```python
from build123d import *

# Parameters (mm, degrees)
F0_R     = 30.022303
F1_DEPTH = 10
F3_DEPTH = 25
F4_R     = 15.13861
F5_DEPTH = 25


with BuildPart() as f1:
    # F0 (on Front) → F1 (new body)
    with BuildSketch(Plane.XZ):
        Circle(F0_R)
    extrude(amount=F1_DEPTH)

    # F2 (on face) → F3 (cut)
    with BuildSketch(Plane.XZ.offset(10)):
        with BuildLine():
            ThreePointArc((-13.51767, 26.806926), (-0.223887, 30.021468), (13.11636, 27.005551))
            ThreePointArc((13.11636, 27.005551), (-0.226298, 30.344822), (-13.51767, 26.806926))
        make_face()
        with BuildLine():
            ThreePointArc((19.663822, -22.686401), (27.429863, -12.524318), (30.022303, 0))
            ThreePointArc((30.022303, 0), (27.31018, -12.469672), (19.663822, -22.686401))
        make_face()
        with BuildLine():
            ThreePointArc((-11.50515, -27.730312), (-22.127404, -20.290802), (-28.62096, -9.065281))
            ThreePointArc((-28.62096, -9.065281), (-22.573017, -20.699429), (-11.50515, -27.730312))
        make_face()
        with BuildLine():
            Line((-8.288842, 15.331867), (-13.51767, 26.806926))
            ThreePointArc((-13.51767, 26.806926), (-27.669836, 11.649842), (-28.62096, -9.065281))
            Line((-28.62096, -9.065281), (-16.901936, -3.498297))
            ThreePointArc((-16.901936, -3.498297), (-15.781932, 7.37434), (-8.288842, 15.331867))
        make_face()
        with BuildLine():
            ThreePointArc((-11.50515, -27.730312), (4.795961, -29.636758), (19.663822, -22.686401))
            Line((19.663822, -22.686401), (11.541307, -13.314021))
            ThreePointArc((11.541307, -13.314021), (3.179849, -16.970197), (-5.885188, -15.918192))
            Line((-5.885188, -15.918192), (-11.50515, -27.730312))
        make_face()
        with BuildLine():
            ThreePointArc((30.022303, 0), (25.44722, 15.930401), (13.11636, 27.005551))
            Line((13.11636, 27.005551), (8.336435, 15.331867))
            ThreePointArc((8.336435, 15.331867), (15.053544, 8.994054), (17.149832, 0))
            Line((17.149832, 0), (30.022303, 0))
        make_face()
    extrude(amount=-F3_DEPTH, mode=Mode.SUBTRACT)

    # F4 (on face) → F5 (cut)
    with BuildSketch(Plane.XZ.offset(10)):
        Circle(F4_R)
    extrude(amount=-F5_DEPTH, mode=Mode.SUBTRACT)


solid = f1.part
```
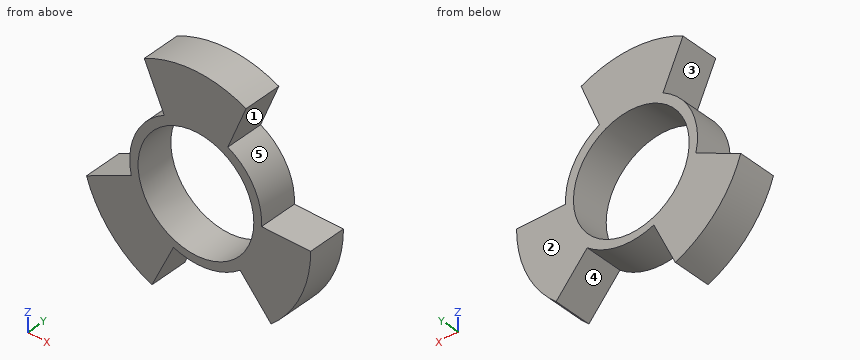
Check sheet for the modelled part. Datum: model origin and axes. Units: mm. Face numbers are marked on the shaded views. A direction names the side the tool comes from. Round coordinates to 2 decimals unless told otherwise and drop trailing zeros. Order: outer loops, then holes, each group sorted by start corner. A loop starts at its lowest first (then second) coordinate and runs counter-clockwise, first axis right, second up. Notation, with made-up numbers: (83.25, 67) -> (94.25, 67) arc R14 ccw to (94.25, 90) -> close; hole circle Ø5 at (-24.75, 15.25). An arc over 180 degrees is marked (long way). One line per item, written item: value. Start each with the question number.
Q1. Cross-section at B-B (x = -7.5). Record the boundary of the cut face in (y, z).
Q2. Cross-section at D-D (x = 0). Record the boundary of the cut face in (y, z).
Q3. Thickness scan on line 1 (Z direction, x = 0, y = -6); line 2 (Z direction, x = 12, y = -6.5); line 3 (X direction, y = -5, z = -3). Record the ranges inside material, lowest first.
Q4. Gauge pin test, flat ends, axial feed: pin 1 Ø2 at (y, z) = (-8.5, -4) entering from +X; pin 2 Ø12 at (x, z) = (22.5, 18.5) entering from +Y; pin 3 Ø3 at (y, z) = (-3, 17) entering from +X; pin 4 Ø1.5 at (y, z) = (-3, -11) entering from +X. Record the tip position at first contact, or that the pin passes through.
Q5. Cross-section at A-A (y = -1.5). Record the boundary of the cut face in (x, z).
Q6. Mould release check, pull along X, two halves, no side actions. Record for the marked faces 3, 4 and 5: pulls with the +X half, pulls with the -X half, needs draft (parallel to the pull), parting line crosses it, or undercut.
Q7. Set-up check for the marked faces 1 and 2: record each of +Z, -Z, +X, -X, +Y, -Y from which the full face is reachable in a straight line by a thin tool's end or side.
Q8. Cross-section at C-C (x = 9). Record the boundary of the cut face in (y, z).
Completed:
1. outline: (-10, -19.31) -> (0, -19.31) -> (0, -13.15) -> (-10, -13.15) -> close; (-10, 13.15) -> (0, 13.15) -> (0, 29.07) -> (-10, 29.07) -> close
2. outline: (-10, -17.15) -> (0, -17.15) -> (0, -15.14) -> (-10, -15.14) -> close; (-10, 15.14) -> (0, 15.14) -> (0, 30.02) -> (-10, 30.02) -> close
3. line 1: z = -17.15 to -15.14, 15.14 to 30.02
3. line 2: z = -13.84 to -9.23, 9.23 to 12.81, 24.28 to 27.52
3. line 3: x = -17.01 to -14.84, 14.84 to 29.87
4. pin 1: stops at x = 29.87
4. pin 2: passes through
4. pin 3: stops at x = 9.63
4. pin 4: stops at x = 28.22
5. outline: (-28.62, -9.07) arc R30.02 ccw to (-11.51, -27.73) -> (-5.89, -15.92) arc R17.49 ccw to (11.54, -13.31) -> (19.66, -22.69) arc R30.02 ccw to (30.02, 0) -> (17.15, 0) arc R16 ccw to (8.34, 15.33) -> (13.12, 27.01) arc R30.02 ccw to (-13.52, 26.81) -> (-8.29, 15.33) arc R17.05 ccw to (-16.9, -3.5) -> close; hole circle Ø30.28 at (0, 0)
6. face 3: pulls with the -X half
6. face 4: undercut
6. face 5: pulls with the +X half
7. face 1: +X, +Y, -Y
7. face 2: +Z, -Z, +X, -X, +Y
8. outline: (-10, -15.01) -> (0, -15.01) -> (0, -12.17) -> (-10, -12.17) -> close; (-10, 12.17) -> (0, 12.17) -> (0, 14.98) -> (-10, 14.98) -> close; (-10, 16.95) -> (0, 16.95) -> (0, 28.64) -> (-10, 28.64) -> close
